Here's how the part is built. I have some questions about the finished solid (model axes, mm). Face numbers are marked on the shaded views. A direction names the side the tool comes from. Coordinates: 2 decimals unless noted, no trailing zeros. Loops run counter-clockwise (first coordinate to the right, second up) from the corner with the lowest first, then second, coordinate; pieces in that order, holes last.
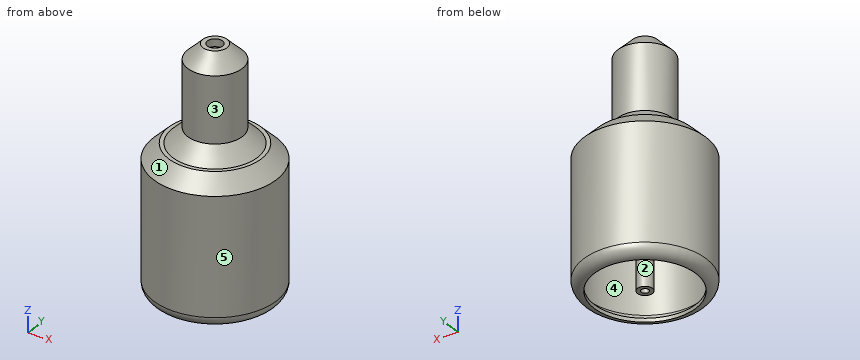
from build123d import *

# Parameters (mm, degrees)
F0_R           = 18.0428144426
F1_DEPTH       = 63.5
F2_W           = 40.2940958738
F2_H           = 94.3237841129
F4_SIZE        = 10
F6_D           = 5
F6_CBORE_D     = 10
F6_CBORE_DEPTH = 5
F7_R           = 7
F8_T           = -2.5


# Not quite as in the source:
# - a shell that OpenCascade refuses in one call is made with other operations: the cavity is built on its own and cut out


with BuildPart() as f1:
    # F0 (on Top) → F1 (new body, symmetric)
    with BuildSketch(Plane.XY):
        Circle(F0_R)
    extrude(amount=F1_DEPTH, both=True)

    # F2 (on Front) → F3 (revolve)
    with BuildSketch(Plane.XZ):
        with Locations((20.4668417573, -47.1034049988)):
            Rectangle(F2_W, F2_H)
    revolve(axis=Axis((0, 0, 0), (0, 0, 1)))

    # F4
    f4_edges = [f1.edges().sort_by_distance(p)[0] for p in [
        (-40.61389, 0, 0.058487),
        (-18.042814, 0, 0.058487),
        (18.042814, 0, 31.779244),
        (-18.042814, 0, 63.5),
    ]]
    chamfer(f4_edges, length=F4_SIZE)

    # F6 (through all)
    with Locations(Plane.XY.offset(63.5)):
        with Locations((0, 0)):
            CounterBoreHole(F6_D / 2, F6_CBORE_D / 2, F6_CBORE_DEPTH)

    # F7
    f7_edges = [f1.edges().sort_by_distance(p)[0] for p in [
        (-40.61389, 0, -94.265297),
    ]]
    fillet(f7_edges, radius=F7_R)

    # F8: a shell. OpenCascade refuses it in one call, so the cavity is built on its own and cut out:
    # the body offset inwards by the wall thickness, plus a prism from it out through each open face.
    f8_core = offset(f1.part, amount=F8_T, kind=Kind.INTERSECTION, mode=Mode.PRIVATE)
    f8_exits = [f8_core.faces().sort_by_distance(p)[0] for p in [
        (-5.950744, 0, -91.765297),
    ]]
    add(f8_core, mode=Mode.SUBTRACT)
    extrude(f8_exits, amount=-F8_T, mode=Mode.SUBTRACT)


solid = f1.part
Q1. Suppose I cut it at A-A on z = -24. Write out the boundary of the cut face in (x, y), and give its area (3 significant figures).
Q2. Will these pins go through, and if not, where does the flat tip stop? P1, Ø2, axis at y = 22.5, z = -39.5, coming from the +X side; P2, Ø2, axis at x = 30, y = -18.5, coming from the +Z side; P3, Ø12, axis at x = -20.5, z = -67.5, coming from the -Y side.
Q3. For the marked faces 3, 4 and 5, which set-ups out of +Z, -Z, +X, -X, +Y, -Y let a thin tool reach every point of the face, with its end or its side?
Q4. We'd pull the mould along Y, two halves only. Please class the marked faces 1 and 2: pulls with the +Y half, pulls with the -Y half, needs draft (parallel to the pull), parting line crosses it, or undercut.
Q5. Please list where these lines run through material, in increasing order: probe 1 along Y at (x, z) = (0, 21); probe 2 along Y at (x, z) = (0, -60); probe 3 along Y at (x, z) = (-3, 23).
Check values:
1. outline: circle Ø81.23 at (0, 0); circle Ø10 at (0, 0); hole circle Ø76.23 at (0, 0); hole circle Ø5 at (0, 0)
1. area: 677 mm2
2. P1: stops at x = 34.46
2. P2: stops at z = -3.57
2. P3: stops at y = -37.94
3. face 3: +Z
3. face 4: none
3. face 5: +Z, -Z
4. face 1: parting line crosses it
4. face 2: undercut
5. probe 1: y = -18.04 to -15.54, -5 to -2.5, 2.5 to 5, 15.54 to 18.04
5. probe 2: y = -40.61 to -38.11, -5 to -2.5, 2.5 to 5, 38.11 to 40.61
5. probe 3: y = -17.79 to -15.25, -4 to 4, 15.25 to 17.79
